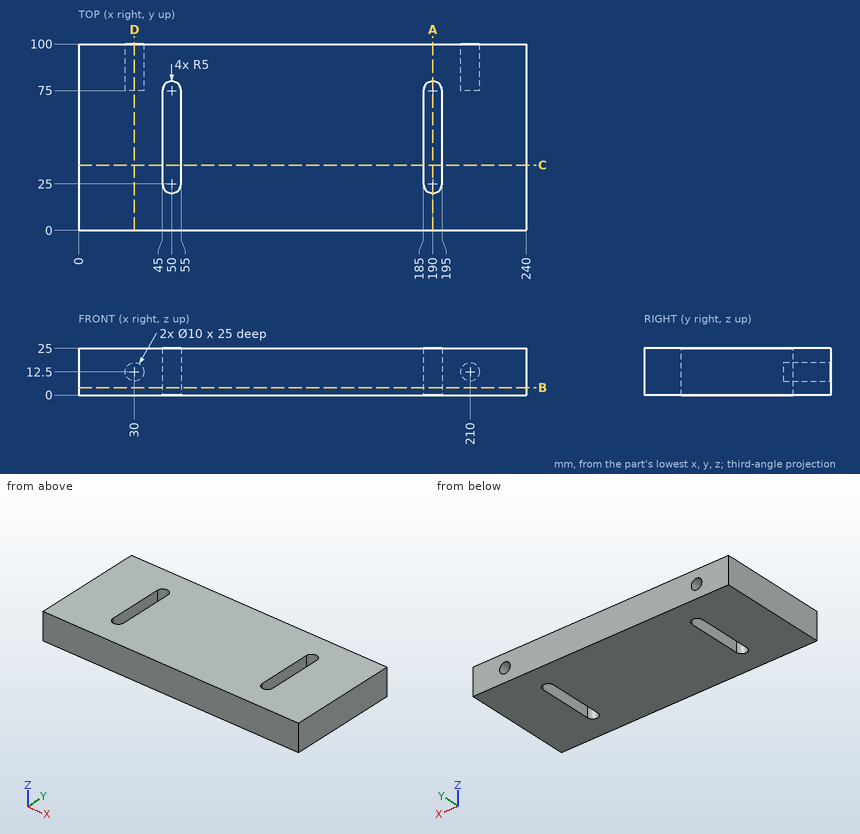
Verification items for this drawing (mm, ordinates from the low corner). Coordinates: 2 decimals unless noted, no trailing zeros. Order: outer loops, then holes, each group sorted by start corner. A loop starts at its lowest first (then second) coordinate and runs counter-clockwise, first axis right, second up. Notation, with made-up numbers: M 27.5,31.25 L 43.5,31.25 A18 ccw 43.5,55.25 Z; hole C 62,50 d4. An arc over 180 degrees is marked long. One line per item, written item: value. Start each with the question number.
Item 1: Sectioned sample at A-A on x = 190. Record the cut outline in (y, z).
Item 2: Sectioned sample at C-C on y = 35. Record the cut outline in (x, z).
Item 3: Thickness scan on probe 1 along X at (y, z) = (81, 12.5); probe 2 along X at (y, z) = (56.5, 8.25); probe 3 along Z at (x, y) = (30, 91). Record the ranges inside material, lowest first.
Item 4: Sectioned sample at B-B on z = 4. Record the cut outline in (x, y).
Item 5: Sectioned sample at D-D on x = 30. Record the cut outline in (y, z).
Calculated:
1. outline: M 0,0 L 20,0 L 20,25 L 0,25 Z; M 80,0 L 100,0 L 100,25 L 80,25 Z
2. outline: M 0,0 L 45,0 L 45,25 L 0,25 Z; M 55,0 L 185,0 L 185,25 L 55,25 Z; M 195,0 L 240,0 L 240,25 L 195,25 Z
3. probe 1: 0 to 25, 35 to 205, 215 to 240
3. probe 2: 0 to 45, 55 to 185, 195 to 240
3. probe 3: 0 to 7.5, 17.5 to 25
4. outline: M 0,0 L 240,0 L 240,100 L 0,100 Z; hole M 45,25 A5 ccw 55,25 L 55,75 A5 ccw 45,75 Z; hole M 185,25 A5 ccw 195,25 L 195,75 A5 ccw 185,75 Z
5. outline: M 0,0 L 100,0 L 100,7.5 L 75,7.5 L 75,17.5 L 100,17.5 L 100,25 L 0,25 Z
